Verification items for the finished model (mm, model axes). A direction names the side the tool comes from. Give positions to 0.01 mm unless a question says otherwise; leave off trailing zeros. Write each loop counter-clockwise with the first axis right and the second up, starting at its lowest first coordinate (ties: lowest second). Pieces come first, ordered by that corner, then holes.
from build123d import *

# Parameters (mm, degrees)
F0_R     = 45
F1_DEPTH = 80
F2_R     = 4
F3_DEPTH = 10
F4_W     = 70
F4_H     = 10
F5_DEPTH = 53.5


with BuildPart() as f1:
    # F0 (on Front) → F1 (new body)
    with BuildSketch(Plane.XZ):
        Polygon((86.916415, 36.896855), (-93.083585, 36.896855), (-67.605668, -33.103145), (-93.083585, -103.103145), (86.916415, -103.103145), (61.438499, -33.103145), align=None)
        with Locations((-3.083585, -33.103145)):
            Circle(F0_R, mode=Mode.SUBTRACT)
    extrude(amount=F1_DEPTH)

    # F2 (on face) → F3 (cut)
    with BuildSketch(Plane(origin=(0, 0, -103.103145), x_dir=(1, 0, 0), z_dir=(0, 0, -1))):
        with Locations((-78.083585, 65)):
            Circle(F2_R)
        with Locations((-78.083585, 15)):
            Circle(F2_R)
        with Locations((71.916415, 15)):
            Circle(F2_R)
        with Locations((71.916415, 65)):
            Circle(F2_R)
    extrude(amount=-F3_DEPTH, mode=Mode.SUBTRACT)

    # F4 (on face) → F5 (cut)
    with BuildSketch(Plane.XY.offset(36.896855)):
        with Locations((-3.083585, -40)):
            Rectangle(F4_W, F4_H)
    extrude(amount=-F5_DEPTH, mode=Mode.SUBTRACT)


solid = f1.part
Item 1: Scan lines: line 1 along Z through (x, y) = (-4.5, -48); line 2 along X through (y, z) = (-15, -98); line 3 along X through (y, z) = (-15.5, -67.5). Record each from-to range of solid material in increasing order.
Answer key:
line 1: z = -103.1 to -78.08, 11.87 to 36.9
line 2: x = -91.23 to -82.08, -74.08 to 67.92, 75.92 to 85.06
line 3: x = -80.13 to -32.1, 25.93 to 73.96
Item 2: Set-up check for faces 1 (the face through (-4, -35, 21)), 2 (the face through (-78, -65, -93.103)), 3 (the face through (74, -39.44, 1.41)), 4 (the face through (-80.166, -39.44, -67.613)): record each of +Z, -Z, +X, -X, +Y, -Y from which the full face is reachable in a straight line by a thin tool's end or side.
Answer key:
face 1: +Z
face 2: -Z
face 3: +X, +Y, -Y
face 4: -X, +Y, -Y
Item 3: Release check for a two-part mould opening along X. For faces 5 (the face through (-4, 0, 15)), 6 (the face through (-80.523, -39.44, 2.387)), 7 (the face through (-12.839, -39.44, -77.033)), 8 (the face through (74.356, -39.44, -68.593)) record: released by +X, released by -X, zero draft, split by the parting line, or undercut.
Answer key:
face 5: zero draft
face 6: released by -X
face 7: undercut
face 8: released by +X
Item 4: Sectioned sample at B-B on z = -23.5. Record the cut outline in (x, y), then the cut area to 3 significant figures.
Answer key:
outline: (-71.1, -80) - (-47.05, -80) - (-47.05, 0) - (-71.1, 0) - close; (40.88, -80) - (64.93, -80) - (64.93, 0) - (40.88, 0) - close
area: 3,850 mm2
Item 5: Sectioned sample at C-C on x = -33. Record the cut outline in (y, z).
Answer key:
outline: (-80, -103.1) - (0, -103.1) - (0, -66.72) - (-80, -66.72) - close; (-80, 0.51) - (-45, 0.51) - (-45, 36.9) - (-80, 36.9) - close; (-35, 0.51) - (0, 0.51) - (0, 36.9) - (-35, 36.9) - close
Item 6: Depth check by flat-ended pin: pin 1 (1.5 mm diameter, centred on y = -59.5, z = -12, fed in from +X); pin 2 (7 mm diameter, centred on x = 71.92, y = -65, fed in from -Z); pin 3 (5 mm diameter, centred on y = -41.5, z = 9.5, fed in from +X). Enter the tip coordinate at first touch or a pass-through.
Answer key:
pin 1: stops at x = 69.39
pin 2: stops at z = -93.1
pin 3: stops at x = 77.85
Item 7: Sectioned sample at A-A on y = -65. Record the cut outline in (x, z).
Answer key:
outline: (-93.08, -103.1) - (-82.08, -103.1) - (-82.08, -93.1) - (-74.08, -93.1) - (-74.08, -103.1) - (67.92, -103.1) - (67.92, -93.1) - (75.92, -93.1) - (75.92, -103.1) - (86.92, -103.1) - (61.44, -33.1) - (86.92, 36.9) - (-93.08, 36.9) - (-67.61, -33.1) - close; hole circle Ø90 at (-3.08, -33.1)
Item 8: Sectioned sample at D-D on z = 26.5. Record the cut outline in (x, y).
Answer key:
outline: (-89.3, -80) - (83.13, -80) - (83.13, 0) - (-89.3, 0) - close; hole (-38.08, -45) - (31.92, -45) - (31.92, -35) - (-38.08, -35) - close
